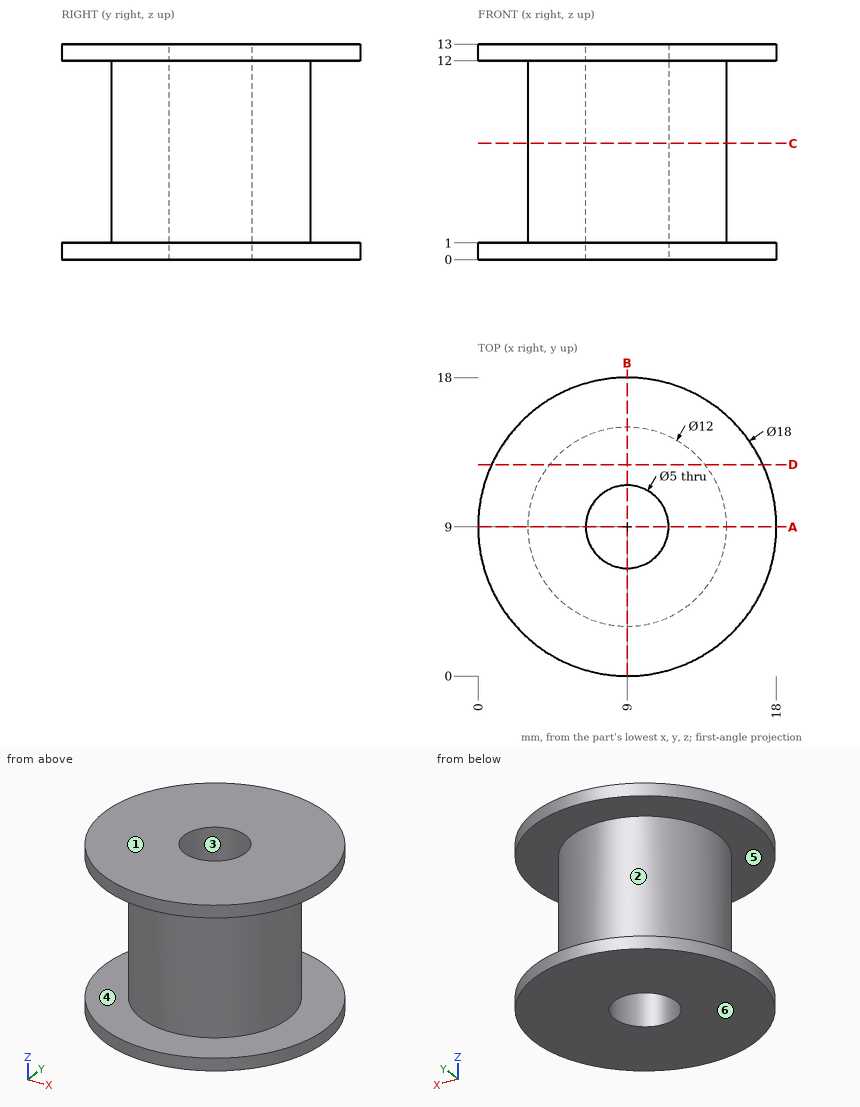
Can you work these out from the drawing? Everything is in mm from the part's minimum corner. A direction names the side the tool comes from. Round coordinates to 2 decimals unless told otherwise and drop trailing zeros. Loops run counter-clockwise (first coordinate to the right, second up) from the corner with the lowest first, then second, coordinate; pieces in that order, holes last. Notation, with made-up numbers: (2, -27) - (17, -27) arc R13 ccw to (17, -6) - close; hole circle Ø7 at (81, 51.25). An arc over 180 degrees is marked (long way). Answer in a Markdown table with one row per item. Add a question column.
Q1. Which directions (+Z, -Z, +X, -X, +Y, -Y) give clear straight access to the entire face, cutting with the end or side of a thin tool? Please do the marked faces 5 and 6.
Q2. For pin 1 Ø5 at (x, y) = (10, 6.5) entering from -Z; pin 2 Ø6 at (x, z) = (11.5, 8.5) entering from +Y; pin 3 Ø4 at (y, z) = (12, 5.5) entering from -X; pin 4 Ø1 at (x, z) = (9, 10.5) entering from -Y, each with a flat end and sliding along its axis, tell me the tip position at first contact or that it passes through.
Q3. I want a section at C-C on z = 7. List the corners of the cut face in (x, y) for me, and give its area (3 significant figures).
Q4. We'd pull the mould along Z, two halves only. Please class the marked faces 1, 2, 3 and 4: pulls with the +Z half, pulls with the -Z half, needs draft (parallel to the pull), parting line crosses it, or undercut.
Q5. I want a section at D-D on y = 12.75. List the corners of the cut face in (x, z) for me.
Q6. I want a section at A-A on y = 9. List the corners of the cut face in (x, z) for me, and give its area (3 significant figures).
Q7. I need wall thicknesses on L1, parallel to Z at x = 2.5, y = 4.5; L2, parallel to Y at x = 9, z = 3; L3, parallel to X at y = 7.25, z = 7.5. Which ranges of each line are inside material? Lowest first, please.
A:
| question | item | result |
|---|---|---|
| 1 | face 5 | none |
| 1 | face 6 | -Z, +X, -X, +Y, -Y |
| 2 | pin 1 | z = 0 |
| 2 | pin 2 | y = 15 |
| 2 | pin 3 | x = 3.08 |
| 2 | pin 4 | y = 3 |
| 3 | outline | circle Ø12 at (9, 9); hole circle Ø5 at (9, 9) |
| 3 | area | 93.5 mm^2 |
| 4 | face 1 | pulls with the +Z half |
| 4 | face 2 | undercut |
| 4 | face 3 | needs draft |
| 4 | face 4 | undercut |
| 5 | outline | (0.82, 0) - (17.18, 0) - (17.18, 1) - (13.68, 1) - (13.68, 12) - (17.18, 12) - (17.18, 13) - (0.82, 13) - (0.82, 12) - (4.32, 12) - (4.32, 1) - (0.82, 1) - close |
| 6 | outline | (0, 0) - (6.5, 0) - (6.5, 13) - (0, 13) - (0, 12) - (3, 12) - (3, 1) - (0, 1) - close; (11.5, 0) - (18, 0) - (18, 1) - (15, 1) - (15, 12) - (18, 12) - (18, 13) - (11.5, 13) - close |
| 6 | area | 103 mm^2 |
| 7 | L1 | 0 to 1, 12 to 13 |
| 7 | L2 | 3 to 6.5, 11.5 to 15 |
| 7 | L3 | 3.26 to 7.21, 10.79 to 14.74 |
